Work out the finished part from the listing and answer in its coordinate system (mm). Face numbers are marked on the shaded views. A direction names the side the tool comes from. Give positions to 0.01 mm unless a question says otherwise; leave off trailing zeros. Order: outer loops, then holes, each group sorted by start corner. A loop starts at its lowest first (then second) coordinate and runs counter-clockwise, first axis right, second up. Notation, with made-up numbers: M 66,70 L 93,70 A15 cw 93,97 Z; hole C -21,56 d7. An arc over 180 degrees is marked long. One line per item, written item: value.
from build123d import *

# Parameters (mm, degrees)
SCHIZZO2_R                     = 67.5
ESTRUSIONE_ESTRUSIONE1_DEPTH   = 5
SCHIZZO3_R                     = 45
ESTRUSIONE_ESTRUSIONE2_DEPTH   = 6
SCHIZZO4_R                     = 26
TAGLIO_ESTRUSIONE1_DEPTH       = 3
SCHIZZO5_R                     = 35
TAGLIO_ESTRUSIONE2_DEPTH       = 9
SMUSSO1_SIZE                   = 1
FORO_PER_VITE_M8_1_D           = 9
FORO_PER_VITE_M8_1_CSINK_D     = 9.05
FORO_PER_VITE_M8_1_CSINK_ANGLE = 90
RIPETIZIONECIRCOLARE1_COUNT    = 6
SCHIZZO9_R                     = 52.5
SCHIZZO9_R_2                   = 49.5
TAGLIO_ESTRUSIONE3_DEPTH       = 1.5
SCHIZZO10_R                    = 45
SCHIZZO10_R_2                  = 41.5
ESTRUSIONE_ESTRUSIONE3_DEPTH   = 4.9
SMUSSO2_SIZE                   = 1


with BuildPart() as part:
    # Schizzo2 → Estrusione-Estrusione1 (new body)
    with BuildSketch(Plane.XY):
        Circle(SCHIZZO2_R)
    extrude(amount=ESTRUSIONE_ESTRUSIONE1_DEPTH)

    # Schizzo3 → Estrusione-Estrusione2 (add)
    with BuildSketch(Plane.XY.offset(5)):
        Circle(SCHIZZO3_R)
    extrude(amount=ESTRUSIONE_ESTRUSIONE2_DEPTH)

    # Schizzo4 → Taglio-Estrusione1 (cut)
    with BuildSketch(Plane(origin=(0, 0, 0), x_dir=(-1, 0, 0), z_dir=(0, 0, -1))):
        Circle(SCHIZZO4_R)
    extrude(amount=-TAGLIO_ESTRUSIONE1_DEPTH, mode=Mode.SUBTRACT)

    # Schizzo5 → Taglio-Estrusione2 (cut, through all)
    with BuildSketch(Plane(origin=(0, 0, 3), x_dir=(-1, 0, 0), z_dir=(0, 0, -1))):
        Circle(SCHIZZO5_R)
    extrude(amount=-TAGLIO_ESTRUSIONE2_DEPTH, mode=Mode.SUBTRACT)

    # Smusso1
    smusso1_edges = [part.edges().sort_by_distance(p)[0] for p in [
        (-67.5, 0, 0),
    ]]
    chamfer(smusso1_edges, length=SMUSSO1_SIZE)

    # Foro per Vite M8-1 (through all)
    with Locations(Plane(origin=(0, 0, 0), x_dir=(-1, 0, 0), z_dir=(0, 0, -1))):
        with Locations((0, 60)):
            foro_per_vite_m8_1 = CounterSinkHole(FORO_PER_VITE_M8_1_D / 2, FORO_PER_VITE_M8_1_CSINK_D / 2, counter_sink_angle=FORO_PER_VITE_M8_1_CSINK_ANGLE)

    # RipetizioneCircolare1: Foro per Vite M8-1 ×6 about axis
    ripetizionecircolare1_axis = Axis((0, 0, 0), (0, 0, 1))
    for i in range(1, RIPETIZIONECIRCOLARE1_COUNT):
        add(foro_per_vite_m8_1.rotate(ripetizionecircolare1_axis, i * 360 / RIPETIZIONECIRCOLARE1_COUNT), mode=Mode.SUBTRACT)

    # Schizzo9 → Taglio-Estrusione3 (cut)
    with BuildSketch(Plane.XY.offset(5)):
        Circle(SCHIZZO9_R)
        Circle(SCHIZZO9_R_2, mode=Mode.SUBTRACT)
    extrude(amount=-TAGLIO_ESTRUSIONE3_DEPTH, mode=Mode.SUBTRACT)

    # Schizzo10 → Estrusione-Estrusione3 (add)
    with BuildSketch(Plane.XY.offset(11)):
        Circle(SCHIZZO10_R)
        Circle(SCHIZZO10_R_2, mode=Mode.SUBTRACT)
    extrude(amount=ESTRUSIONE_ESTRUSIONE3_DEPTH)

    # Smusso2
    smusso2_edges = [part.edges().sort_by_distance(p)[0] for p in [
        (-45, 0, 15.9),
    ]]
    chamfer(smusso2_edges, length=SMUSSO2_SIZE)


solid = part.part
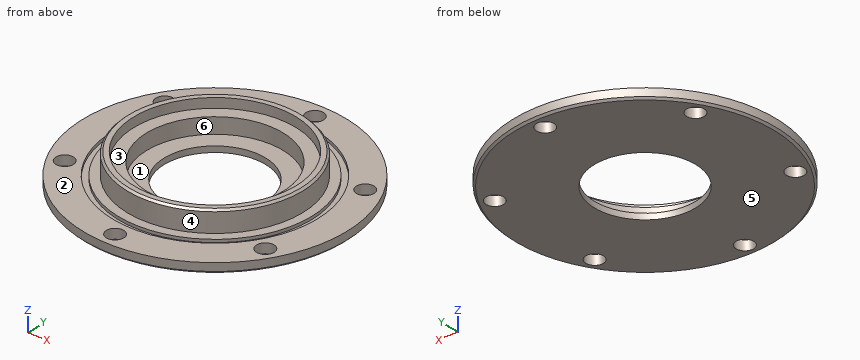
(1) Find the intervals of material crossed by probe 1 along Y at (x, z) = (1.5, 9.5) (3 decimals); probe 2 along Y at (x, z) = (51.5, 1.5); probe 3 along X at (y, z) = (3.5, 4), in increasing order. Write a range as from..to.
Findings:
probe 1: y = -44.975..-34.968, 34.968..44.975
probe 2: y = -43.63..-34.48, -25.52..25.52, 34.48..43.63
probe 3: x = -67.41..-52.38, -49.38..-34.82, 34.82..49.38, 52.38..67.41
(2) Section C-C, the plane x = 0 is taken. Give the number of separate pieces and of enclosed holes in the cut face, then the cut area to 3 significant figures.
Findings:
separate pieces: 4
enclosed holes: 0
area: 432 mm^2
(3) Determine the mould class of the marked faces 1, 2, 3 and 4 for opening direction Y: pulls with the +Y half, pulls with the -Y half, needs draft (parallel to the pull), parting line crosses it, or undercut.
Findings:
face 1: undercut
face 2: needs draft
face 3: undercut
face 4: parting line crosses it
(4) Which of the six approach directions +Z, -Z, +X, -X, +Y, -Y give full straight-line access (tool end or side, diameter ignored) to the marked faces 5 and 6?
Findings:
face 5: -Z, +X, -X, +Y, -Y
face 6: +Z
(5) Section B-B, the plane z = 13 is taken. Give the vertices of the cut face in (x, y).
Findings:
outline: C 0,0 d90; hole C 0,0 d83
(6) Given P1, Ø7, axis at x = 0, y = -60, coming from the -Z side; P2, Ø1, axis at x = -10, z = 12, coming from the +Y side; P3, Ø11.5, axis at x = 0, y = 60, coming from the +Z side; P4, Ø5, axis at x = -26, z = 13.5, coming from the -Y side, each flat-ended and moving along its own axis, determine where each tip first touches the part or whether it passes through.
Findings:
P1: passes through
P2: stops at y = 43.99
P3: stops at z = 5
P4: stops at y = -38.38
